Solid Edge part; units mm, degrees
sketch "Sketch1" plane through (0, 0, 0) normal (0, -1, 0) x (1, 0, 0)
  line L0 (0.1071, -0.1481) -> (0.1071, 2.6019)
  line L1 (4.1071, 2.4819) -> (0.1071, 2.6019)
  line L2 (4.1071, 2.4819) -> (4.1071, 2.1019)
  line L3 (4.1071, 2.1019) -> (24.6071, 1.6019)
  line L4 (24.6071, -0.1481) -> (24.6071, 1.6019)
revolve "RevolvedProtrusion1" add sketch "Sketch1" angle 360 about axis through (0.1071, 0, -0.1481) along (1, 0, 0)
sketch "Sketch2" plane through (24.7552, 0, 0) normal (0, 0, 1) x (0, 1, 0)
  line L0 (1.6556, -3.3861) -> (1.7437, 0.1481)
  line L1 (1.7437, 0.1481) -> (-1.7437, 0.1481)
  line L2 (-1.7437, 0.1481) -> (-1.6556, -3.4668)
  arc A0 (-1.6556, -3.4668) -> (1.6556, -3.3861) centre (0, -3.4265) ccw
extrude "ExtrudedProtrusion_2" add sketch "Sketch2" along normal mid plane 2
sketch "Sketch3" plane through (27.2224, 0, -0.1481) normal (0, 0, 1) x (-0.9997, -0.0244, 0)
  line L0 (-3.4837, -2.415) -> (2.572, -2.5627)
  line L1 (2.572, -2.5627) -> (2.572, -1.807)
  line L2 (2.572, -1.807) -> (-3.4837, -1.6593)
  line L3 (-3.4837, -1.6593) -> (-3.4837, -2.415)
revolve "RevolvedCutout1" cut sketch "Sketch3" angle 360 about axis through (24.6071, 0, -0.1481) along (1, 0, 0)
sketch "Sketch4" plane through (27.2224, 0, -1) normal (0, 0, -1) x (0, 1, 0)
  circle A0 centre (0, 0.9592) radius 0.95
extrude "Cutout1" cut sketch "Sketch4" against normal up to vertex (2 mm away)
sketch "Sketch5" plane through (0.1071, 0, -0.1481) normal (-1, 0, 0) x (0, 0, -1)
  circle A0 centre (-0.1481, 0) radius 1
extrude "ExtrudedCutout_2" cut sketch "Sketch5" against normal blind 15
properties material "Stainless Steel, 420"
Geometry: final body of the model. Coordinates: model frame, mm. A direction names the side the tool comes from. Give positions to 0.01 mm unless a question says otherwise; leave off trailing zeros. Write each loop counter-clockwise with the first axis right and the second up, starting at its lowest first coordinate (ties: lowest second). Pieces come first, ordered by that corner, then holes. Notation, with made-up numbers: (28.5, 68.5) -> (58.5, 68.5) arc R15 cw to (58.5, 93.5) -> close; hole circle Ø4 at (79, -37). An arc over 180 degrees is marked (long way). Answer as a JSON object with one key per item and string values.
1. Contact query for flat-ended pins moving along their axis: pin 1 (1 mm diameter, centred on y = 0, z = 0, fed in from -X); pin 2 (2 mm diameter, centred on x = 27, y = 0.5, fed in from +Z); pin 3 (1.5 mm diameter, centred on x = 27.5, y = 0.5, fed in from -Z); pin 4 (1.1 mm diameter, centred on x = 28.18, y = 0, fed in from +Z). Output: stop coordinate, or through.
Ans:
{"pin 1": "stops at x = 15.11", "pin 2": "stops at z = 1", "pin 3": "stops at z = -1", "pin 4": "passes through"}
2. Ray query, probe 1 along Y at (x, z) = (3.75, 0); probe 2 along X at (y, z) = (0, 0.45); probe 3 along X at (y, z) = (-2.45, 0.4). Return the intervals inside material, ascending. Write a range as from..to.
Ans:
{"probe 1": "y = -2.64..-1, 1..2.64", "probe 2": "x = 15.11..27.23, 29.13..29.84", "probe 3": "x = 0.11..4.11"}
3. Access query for faces 1 (the conical face through (2.08, -1.64, -2.28)), 2 (the flat face through (15.107, 0, 0)), 3 (the flat face through (24.607, 0, -1.4)), 4 (the flat face through (27, 0, 1)). Directions: +Z, -Z, +X, -X, +Y, -Y. A direction counts if a zero-diameter tool reaches every point of the face in a straight line with its end or side. Return the directions, or none.
Ans:
{"face 1": "+X", "face 2": "-X", "face 3": "-Z, +X, +Y, -Y", "face 4": "+Z, +X, +Y, -Y"}
4. Cut plane B-B on x = 24. Output: boundary loops of the cut face in (y, z), and give its area (3 significant figures).
Ans:
{"outline": "circle Ø3.53 at (0, -0.15)", "area": "9.78 mm^2"}
5. Mould query, pull axis Y, two halves, no side actions, for faces 5 (the cylindrical face through (29.836, 0.077, -0.014)), 6 (the cylindrical face through (29.124, -0.124, -0.014)), 7 (the flat face through (27, 0, -1)). Classes: pulls with the +Y half, pulls with the -Y half, needs draft (parallel to the pull), parting line crosses it, or undercut.
Ans:
{"face 5": "parting line crosses it", "face 6": "undercut", "face 7": "needs draft"}
